For this review, take the finished solid that the model builds, in its own axes (mm). A direction names the side the tool comes from. Give positions to 0.01 mm unless a question says otherwise; leave off trailing zeros. Write each loop counter-clockwise with the first axis right and the second up, starting at its lowest first coordinate (ties: lowest second). Pieces come first, ordered by that corner, then holes.
1) We need section B-B on z = -9.5. Give the number of separate pieces and of enclosed holes in the cut face, and give its area (3 significant figures).
2) Wall thickness on line 1 along Y through (x, z) = (-3.55, 0); line 2 along Z through (x, y) = (-12, -4); line 3 along X through (y, z) = (-21, 8.8): over which ranges is each line inside the solid? List them lowest first.
3) For P1, Ø16, axis at x = 1, y = -21.5, coming from the -Z side; P2, Ø6, axis at x = -2, z = 1.5, coming from the -Y side; P3, Ø10, axis at y = -25.5, z = -2, coming from the -X side; P4, Ø5, axis at y = -21, z = 0, coming from the +X side, all flat-tipped, find the tip position at first contact; note any pin that passes through.
4) Machinability: for faces 1 (the face through (-3, -27, 1)), 2 (the face through (3, -15, 1)), 3 (the face through (-14.74, -7.48, 19.09)), which of the approach directions +Z, -Z, +X, -X, +Y, -Y give a long, thin tool a straight path to every point of the face, cutting with its end or side? Answer none if there is none.
5) Draft analysis for pull direction Z (two halves, no side actions). For faces 4 (the face through (5, -28, 11)), 5 (the face through (15.202, -35.985, 0.66)), 6 (the face through (-2.21, -25.46, 2.03)), 7 (the face through (-13, -5, -21)), state which applies: pulls with the +Z half, pulls with the -Z half, needs draft (parallel to the pull), parting line crosses it, or undercut.
6) We need section A-A on y = -38.5. Give the boundary of the cut face in (x, z), and give its area (3 significant figures).
from build123d import *

# Parameters (mm, degrees)
F0_W      = 42
F0_H      = 42
F0_R      = 3
F1_DEPTH  = 42
F2_R      = 20
F2_R_2    = 15
F3_DEPTH  = 5
F2_R_3    = 8
F4_DEPTH  = 10
F2_R_4    = 3
F5_DEPTH  = 15
F6_R      = 20
F6_R_2    = 15
F7_DEPTH  = 5
F6_R_3    = 8
F8_DEPTH  = 10
F6_R_4    = 3
F9_DEPTH  = 15
F10_DEPTH = 42
F11_R     = 20
F11_R_2   = 15
F12_DEPTH = 5
F11_R_3   = 8
F13_DEPTH = 10
F11_R_4   = 3
F14_DEPTH = 15
F15_R     = 20
F15_R_2   = 15
F16_DEPTH = 5
F15_R_3   = 8
F17_DEPTH = 10
F15_R_4   = 3
F18_DEPTH = 15
F19_R     = 20
F19_R_2   = 15
F20_DEPTH = 5
F19_R_3   = 8
F21_DEPTH = 10
F19_R_4   = 3
F22_DEPTH = 15
F23_DEPTH = 42
F24_R     = 20
F24_R_2   = 15
F25_DEPTH = 5
F24_R_3   = 8
F26_DEPTH = 10
F24_R_4   = 3
F27_DEPTH = 15


with BuildPart() as f1:
    # F0 (on Front) → F1 (new body)
    with BuildSketch(Plane.XZ):
        Rectangle(F0_W, F0_H)
        Circle(F0_R, mode=Mode.SUBTRACT)
    extrude(amount=F1_DEPTH)

    # F2 (on face) → F3 (cut)
    with BuildSketch(Plane.XZ.offset(42)):
        Circle(F2_R)
        Circle(F2_R_2, mode=Mode.SUBTRACT)
    extrude(amount=-F3_DEPTH, mode=Mode.SUBTRACT)

    # F2 (on face) → F4 (cut)
    with BuildSketch(Plane.XZ.offset(42)):
        Circle(F2_R_2)
        Circle(F2_R_3, mode=Mode.SUBTRACT)
    extrude(amount=-F4_DEPTH, mode=Mode.SUBTRACT)

    # F2 (on face) → F5 (cut)
    with BuildSketch(Plane.XZ.offset(42)):
        Circle(F2_R_3)
        Circle(F2_R_4, mode=Mode.SUBTRACT)
    extrude(amount=-F5_DEPTH, mode=Mode.SUBTRACT)

    # F6 (on face) → F7 (cut)
    with BuildSketch(Plane(origin=(-21, 0, 0), x_dir=(0, -1, 0), z_dir=(-1, 0, 0))):
        with Locations((21, 0)):
            Circle(F6_R)
        with Locations((21, 0)):
            Circle(F6_R_2, mode=Mode.SUBTRACT)
    extrude(amount=-F7_DEPTH, mode=Mode.SUBTRACT)

    # F6 (on face) → F8 (cut)
    with BuildSketch(Plane(origin=(-21, 0, 0), x_dir=(0, -1, 0), z_dir=(-1, 0, 0))):
        with Locations((21, 0)):
            Circle(F6_R_2)
        with Locations((21, 0)):
            Circle(F6_R_3, mode=Mode.SUBTRACT)
    extrude(amount=-F8_DEPTH, mode=Mode.SUBTRACT)

    # F6 (on face) → F9 (cut)
    with BuildSketch(Plane(origin=(-21, 0, 0), x_dir=(0, -1, 0), z_dir=(-1, 0, 0))):
        with Locations((21, 0)):
            Circle(F6_R_3)
        with Locations((21, 0)):
            Circle(F6_R_4, mode=Mode.SUBTRACT)
    extrude(amount=-F9_DEPTH, mode=Mode.SUBTRACT)

    # F6 (on face) → F10 (cut)
    with BuildSketch(Plane(origin=(-21, 0, 0), x_dir=(0, -1, 0), z_dir=(-1, 0, 0))):
        with Locations((21, 0)):
            Circle(F6_R_4)
    extrude(amount=-F10_DEPTH, mode=Mode.SUBTRACT)

    # F11 (on face) → F12 (cut)
    with BuildSketch(Plane(origin=(0, 0, 0), x_dir=(-1, 0, 0), z_dir=(0, 1, 0))):
        Circle(F11_R)
        Circle(F11_R_2, mode=Mode.SUBTRACT)
    extrude(amount=-F12_DEPTH, mode=Mode.SUBTRACT)

    # F11 (on face) → F13 (cut)
    with BuildSketch(Plane(origin=(0, 0, 0), x_dir=(-1, 0, 0), z_dir=(0, 1, 0))):
        Circle(F11_R_2)
        Circle(F11_R_3, mode=Mode.SUBTRACT)
    extrude(amount=-F13_DEPTH, mode=Mode.SUBTRACT)

    # F11 (on face) → F14 (cut)
    with BuildSketch(Plane(origin=(0, 0, 0), x_dir=(-1, 0, 0), z_dir=(0, 1, 0))):
        Circle(F11_R_3)
        Circle(F11_R_4, mode=Mode.SUBTRACT)
    extrude(amount=-F14_DEPTH, mode=Mode.SUBTRACT)

    # F15 (on face) → F16 (cut)
    with BuildSketch(Plane.YZ.offset(21)):
        with Locations((-21, 0)):
            Circle(F15_R)
        with Locations((-21, 0)):
            Circle(F15_R_2, mode=Mode.SUBTRACT)
    extrude(amount=-F16_DEPTH, mode=Mode.SUBTRACT)

    # F15 (on face) → F17 (cut)
    with BuildSketch(Plane.YZ.offset(21)):
        with Locations((-21, 0)):
            Circle(F15_R_2)
        with Locations((-21, 0)):
            Circle(F15_R_3, mode=Mode.SUBTRACT)
    extrude(amount=-F17_DEPTH, mode=Mode.SUBTRACT)

    # F15 (on face) → F18 (cut)
    with BuildSketch(Plane.YZ.offset(21)):
        with Locations((-21, 0)):
            Circle(F15_R_3)
        with Locations((-21, 0)):
            Circle(F15_R_4, mode=Mode.SUBTRACT)
    extrude(amount=-F18_DEPTH, mode=Mode.SUBTRACT)

    # F19 (on face) → F20 (cut)
    with BuildSketch(Plane.XY.offset(21)):
        with Locations((0, -21)):
            Circle(F19_R)
        with Locations((0, -21)):
            Circle(F19_R_2, mode=Mode.SUBTRACT)
    extrude(amount=-F20_DEPTH, mode=Mode.SUBTRACT)

    # F19 (on face) → F21 (cut)
    with BuildSketch(Plane.XY.offset(21)):
        with Locations((0, -21)):
            Circle(F19_R_2)
        with Locations((0, -21)):
            Circle(F19_R_3, mode=Mode.SUBTRACT)
    extrude(amount=-F21_DEPTH, mode=Mode.SUBTRACT)

    # F19 (on face) → F22 (cut)
    with BuildSketch(Plane.XY.offset(21)):
        with Locations((0, -21)):
            Circle(F19_R_3)
        with Locations((0, -21)):
            Circle(F19_R_4, mode=Mode.SUBTRACT)
    extrude(amount=-F22_DEPTH, mode=Mode.SUBTRACT)

    # F19 (on face) → F23 (cut)
    with BuildSketch(Plane.XY.offset(21)):
        with Locations((0, -21)):
            Circle(F19_R_4)
    extrude(amount=-F23_DEPTH, mode=Mode.SUBTRACT)

    # F24 (on face) → F25 (cut)
    with BuildSketch(Plane(origin=(0, 0, -21), x_dir=(1, 0, 0), z_dir=(0, 0, -1))):
        with Locations((0, 21)):
            Circle(F24_R)
        with Locations((0, 21)):
            Circle(F24_R_2, mode=Mode.SUBTRACT)
    extrude(amount=-F25_DEPTH, mode=Mode.SUBTRACT)

    # F24 (on face) → F26 (cut)
    with BuildSketch(Plane(origin=(0, 0, -21), x_dir=(1, 0, 0), z_dir=(0, 0, -1))):
        with Locations((0, 21)):
            Circle(F24_R_2)
        with Locations((0, 21)):
            Circle(F24_R_3, mode=Mode.SUBTRACT)
    extrude(amount=-F26_DEPTH, mode=Mode.SUBTRACT)

    # F24 (on face) → F27 (cut)
    with BuildSketch(Plane(origin=(0, 0, -21), x_dir=(1, 0, 0), z_dir=(0, 0, -1))):
        with Locations((0, 21)):
            Circle(F24_R_3)
        with Locations((0, 21)):
            Circle(F24_R_4, mode=Mode.SUBTRACT)
    extrude(amount=-F27_DEPTH, mode=Mode.SUBTRACT)


solid = f1.part
Results list:
1. separate pieces: 9
1. enclosed holes: 1
1. area: 406 mm2
2. line 1: y = -27 to -24, -18 to -15
2. line 2: z = -21 to -16, 16 to 21
2. line 3: x = -11 to -8, 8 to 11
3. P1: stops at z = -11
3. P2: stops at y = -27
3. P3: stops at x = -11
3. P4: passes through
4. face 1: -Y
4. face 2: +Y
4. face 3: +Z
5. face 4: pulls with the +Z half
5. face 5: undercut
5. face 6: undercut
5. face 7: pulls with the -Z half
6. outline: (-21, -21) - (-9.68, -21) - (-9.68, -17.5) arc R20 cw to (-17.5, -9.68) - (-21, -9.68) - close; (-21, 9.68) - (-17.5, 9.68) arc R20 cw to (-9.68, 17.5) - (-9.68, 21) - (-21, 21) - close; (9.68, -21) - (21, -21) - (21, -9.68) - (17.5, -9.68) arc R20 cw to (9.68, -17.5) - close; (9.68, 17.5) arc R20 cw to (17.5, 9.68) - (21, 9.68) - (21, 21) - (9.68, 21) - close
6. area: 367 mm2
